Geometry: see drawing. Coordinates: mm, zero at the bounding-box minimum. A direction names the side the tool comes from. Round coordinates to 2 decimals unless told otherwise and drop trailing zeros. Order: outer loops, then holes, each group sorted by start corner. A loop starts at its lowest first (then second) coordinate and runs counter-clockwise, first axis right, second up. Notation, with made-up numbers: (85.25, 73) -> (107.25, 73) arc R15 ccw to (107.25, 95) -> close; hole circle Ø10 at (24.25, 82.5). An arc over 180 degrees is marked (long way). Use a Markdown table: item, result.
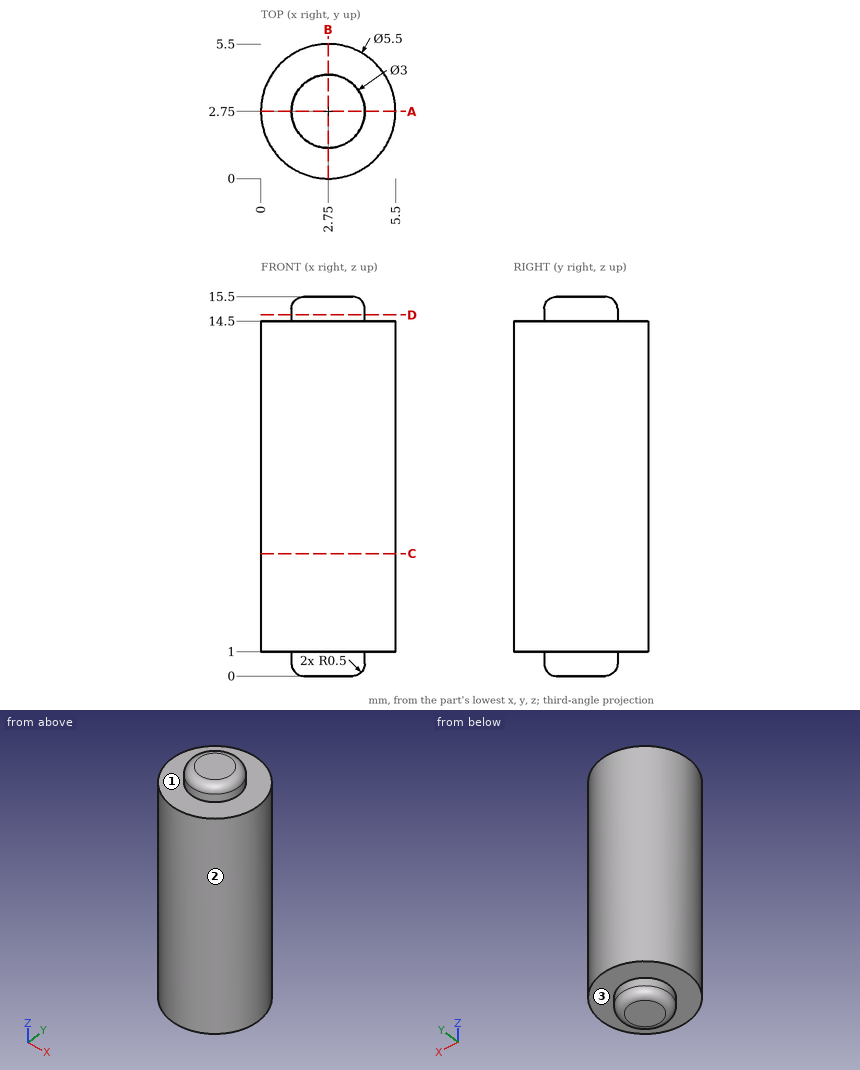
1) Cut plane A-A on y = 2.75. Return loops of the section in (x, z), and give its area (3 significant figures).
Answer key:
| item | result |
|---|---|
| outline | (0, 1) -> (1.25, 1) -> (1.25, 0.5) arc R0.5 ccw to (1.75, 0) -> (3.75, 0) arc R0.5 ccw to (4.25, 0.5) -> (4.25, 1) -> (5.5, 1) -> (5.5, 14.5) -> (4.25, 14.5) -> (4.25, 15) arc R0.5 ccw to (3.75, 15.5) -> (1.75, 15.5) arc R0.5 ccw to (1.25, 15) -> (1.25, 14.5) -> (0, 14.5) -> close |
| area | 80.0 mm^2 |
2) Set-up query: the marked faces 1, 2 and 3. Return all of +Z, -Z, +X, -X, +Y, -Y with unobstructed straight access to the full face (end or side cutting, diameter ignored); none if empty.
Answer key:
| item | result |
|---|---|
| face 1 | +Z |
| face 2 | +Z, -Z |
| face 3 | -Z |
3) Contact query for a flat-ended pin moving along its axis: P1, Ø1.5, axis at y = 1, z = 7.5, coming from the +X side. Output: stop coordinate, or through.
Answer key:
| item | result |
|---|---|
| P1 | stops at x = 5.31 |
4) Ray query, probe 1 along Z at (x, y) = (3.2, 4.65); probe 2 along Y at (x, z) = (2.6, 12.75); probe 3 along X at (y, z) = (4.9, 4). Return the intervals inside material, ascending.
Answer key:
| item | result |
|---|---|
| probe 1 | z = 1 to 14.5 |
| probe 2 | y = 0 to 5.5 |
| probe 3 | x = 1.04 to 4.46 |
5) Cut plane D-D on z = 14.75. Return loops of the section in (x, y).
Answer key:
| item | result |
|---|---|
| outline | circle Ø3 at (2.75, 2.75) |
6) Cut plane C-C on z = 5. Return loops of the section in (x, y).
Answer key:
| item | result |
|---|---|
| outline | circle Ø5.5 at (2.75, 2.75) |
